from build123d import *

# Parameters (mm, degrees)
SKETCH_1_W      = 30
SKETCH_1_H      = 30
SKETCH_1_R      = 1.5
EXTRUDE_1_DEPTH = 2.5
SKETCH_2_R      = 13
EXTRUDE_2_DEPTH = 3
REVOLVE_1_ANGLE = 180


with BuildPart() as part:
    # Эскиз1 → Бобышка-Вытянуть1 (new body)
    with BuildSketch(Plane(origin=(0, 0, 0), x_dir=(1, 0, 0), z_dir=(0, 1, 0))):
        Rectangle(SKETCH_1_W, SKETCH_1_H)
        with Locations(Location((-12.5, 12.5, 0), (0, 0, 270))):
            Circle(SKETCH_1_R, mode=Mode.SUBTRACT)
        with Locations(Location((12.5, 12.5, 0), (0, 0, 270))):
            Circle(SKETCH_1_R, mode=Mode.SUBTRACT)
        with Locations(Location((-12.5, -12.5, 0), (0, 0, 270))):
            Circle(SKETCH_1_R, mode=Mode.SUBTRACT)
        with Locations(Location((12.5, -12.5, 0), (0, 0, 270))):
            Circle(SKETCH_1_R, mode=Mode.SUBTRACT)
    extrude(amount=EXTRUDE_1_DEPTH)

    # Эскиз2 → Бобышка-Вытянуть2 (add)
    with BuildSketch(Plane(origin=(0, 2.5, 0), x_dir=(1, 0, 0), z_dir=(0, 1, 0))):
        with Locations(Location((0, 0, 0), (0, 0, 270))):
            Circle(SKETCH_2_R)
    extrude(amount=EXTRUDE_2_DEPTH)

    # Эскиз3 → Повернуть1 (revolve)
    with BuildSketch(Plane(origin=(0, 5.5, 0), x_dir=(1, 0, 0), z_dir=(0, 1, 0))):
        with BuildLine():
            Line((0, 13), (0, -13))
            ThreePointArc((0, -13), (-13, 0), (0, 13))
        make_face()
    revolve(axis=Axis((0, 5.5, -13), (0, 0, -1)), revolution_arc=REVOLVE_1_ANGLE)


solid = part.part
Verification items for the finished model (mm, model axes). A direction names the side the tool comes from. Coordinates: 2 decimals unless noted, no trailing zeros. Order: outer loops, then holes, each group sorted by start corner. A loop starts at its lowest first (then second) coordinate and runs counter-clockwise, first axis right, second up.
Item 1: Section check B-B, the plane x = 0. Enter the section's corners in (y, z).
Filled in:
outline: (0, -15) - (2.5, -15) - (2.5, -13) - (5.5, -13) arc R13 ccw to (5.5, 13) - (2.5, 13) - (2.5, 15) - (0, 15) - close
Item 2: Release check for a two-part mould opening along Z. For faces 1 (the face through (-12.43, 1.23, -14)), 2 (the face through (15, 1, 0)), 3 (the face through (0, 1, 15)), 4 (the face through (-7.91, 3.979, -10.316)) record: +Z half, -Z half, draft (parallel to the pull), parting line (faces both ways), or undercut.
Filled in:
face 1: undercut
face 2: draft
face 3: +Z half
face 4: parting line
Item 3: Access from +Z, -Z, +X, -X, +Y, -Y to the whole of each face (thin tool, end or side, straight path). Record for faces 5 (the face through (-14, 2.5, 0)), 6 (the face through (0, 0, 0)).
Filled in:
face 5: +Y
face 6: +Z, -Z, +X, -X, -Y
Item 4: Section check D-D, the plane z = -1.25. Enter the section's corners in (x, y), then the cut area to 3 significant figures.
Filled in:
outline: (-15, 0) - (15, 0) - (15, 2.5) - (12.94, 2.5) - (12.94, 5.5) arc R12.94 ccw to (-12.94, 5.5) - (-12.94, 2.5) - (-15, 2.5) - close
area: 416 mm2
Item 5: Material ranges on L1, parallel to X at y = 1.25, z = 12.5; L2, parallel to Z at x = 11.75, y = 1.5; L3, parallel to Y at x = 8.75, z = -10.75, recorded low to high.
Filled in:
L1: x = -15 to -14, -11 to 11, 14 to 15
L2: z = -15 to -13.8, -11.2 to 11.2, 13.8 to 15
L3: y = 0 to 2.5
Item 6: Section check A-A, the plane z = 11.75. Enter the section's corners in (x, y), then the cut area to 3 significant figures.
Filled in:
outline: (-15, 0) - (-13.8, 0) - (-13.8, 2.5) - (-15, 2.5) - close; (-11.2, 0) - (11.2, 0) - (11.2, 2.5) - (5.56, 2.5) - (5.56, 5.5) arc R5.56 ccw to (-5.56, 5.5) - (-5.56, 2.5) - (-11.2, 2.5) - close; (13.8, 0) - (15, 0) - (15, 2.5) - (13.8, 2.5) - close
area: 144 mm2
Item 7: Section check C-C, the plane x = -12.5. Enter the section's corners in (y, z), then the cut area to 3 significant figures.
Filled in:
outline: (0, -15) - (2.5, -15) - (2.5, -14) - (0, -14) - close; (0, -11) - (2.5, -11) - (2.5, -3.57) - (5.5, -3.57) arc R3.57 ccw to (5.5, 3.57) - (2.5, 3.57) - (2.5, 11) - (0, 11) - close; (0, 14) - (2.5, 14) - (2.5, 15) - (0, 15) - close
area: 101 mm2
Item 8: Depth check by flat-ended pin: pin 1 (15 mm diameter, centred on x = 2.5, z = 3.5, fed in from +Y); pin 2 (6 mm diameter, centred on x = 4, z = 7.5, fed in from +Y); pin 3 (8 mm diameter, centred on x = 11, z = -5.5, fed in from +Y). Enter the tip coordinate at first touch or a pass-through.
Filled in:
pin 1: stops at y = 18.5
pin 2: stops at y = 17.28
pin 3: stops at y = 15.51
